from build123d import *

# Parameters (mm, degrees)
BOSS_EXTRUDE1_DEPTH = 2
CUT_EXTRUDE1_DEPTH  = 103
CUT_EXTRUDE2_DEPTH  = 103
SKETCH8_W           = 494.939291997
SKETCH8_H           = 36.91417239
CUT_EXTRUDE3_DEPTH  = 103
SKETCH9_W           = 80
SKETCH9_H           = 22
CUT_EXTRUDE4_DEPTH  = 103
SKETCH10_W          = 80
SKETCH10_H          = 22
CUT_EXTRUDE5_DEPTH  = 10
CUT_EXTRUDE26_DEPTH = 50
SKETCH20_W          = 123.508554763
SKETCH20_H          = 186.038500142
CUT_EXTRUDE27_DEPTH = 50


with BuildPart() as part:
    # Sketch4 → Boss-Extrude1 (new body)
    with BuildSketch(Plane.XY):
        Polygon((-808.497250172, 502.106800376), (-261.98073047, 502.105226222), (-261.98073047, 480.770733626), (-232.677404129, 480.770733626), (-232.677404129, 452.134951617), (-212.25184889, 452.134951617), (-212.192076558, 346.868854324), (-232.677404129, 346.868854324), (-232.677404129, 295.854721303), (-216.917061767, 295.854721303), (-311.499917796, 132.032409135), (-368.546557809, 132.032409135), (-368.546557809, 112.12343356), (-705.513477189, 112.12343356), (-705.513477189, 132.032409135), (-763.511495449, 132.032409135), (-858.513561886, 295.854721303), (-842.744632695, 296.076779874), (-842.744632695, 346.305423028), (-862.968217561, 346.305423028), (-862.968217561, 452.932027611), (-841.983456779, 452.932027611), (-841.983456779, 482.016653843), (-813.304156304, 482.016653843), (-808.497250172, 482.016653843), align=None)
    extrude(amount=BOSS_EXTRUDE1_DEPTH)

    # Sketch6 → Cut-Extrude1 (cut)
    with BuildSketch(Plane.XY.offset(2)):
        Polygon((-822.786730896, 234.247092346), (-802.890229544, 245.785256582), (-762.757484374, 176.580034487), (-782.653985726, 165.041870251), align=None)
    extrude(amount=-CUT_EXTRUDE1_DEPTH, mode=Mode.SUBTRACT)

    # Sketch7 → Cut-Extrude2 (cut)
    with BuildSketch(Plane(origin=(0, 0, 0), x_dir=(-1, 0, 0), z_dir=(0, 0, -1))):
        Polygon((245.988579257, 245.501375956), (264.175112736, 256.001375956), (304.175112736, 186.719343654), (285.988579257, 176.219343654), align=None)
    extrude(amount=-CUT_EXTRUDE2_DEPTH, mode=Mode.SUBTRACT)

    # Sketch8 → Cut-Extrude3 (cut)
    with BuildSketch(Plane.XY.offset(2)):
        with Locations((-533.868102369, 451.361565469)):
            Rectangle(SKETCH8_W, SKETCH8_H)
    extrude(amount=-CUT_EXTRUDE3_DEPTH, mode=Mode.SUBTRACT)

    # Sketch9 → Cut-Extrude4 (cut)
    with BuildSketch(Plane(origin=(0, 0, 0), x_dir=(-1, 0, 0), z_dir=(0, 0, -1))):
        with Locations((427.942047779, 123.12343356)):
            Rectangle(SKETCH9_W, SKETCH9_H)
    extrude(amount=-CUT_EXTRUDE4_DEPTH, mode=Mode.SUBTRACT)

    # Sketch10 → Cut-Extrude5 (cut)
    with BuildSketch(Plane(origin=(0, 0, 0), x_dir=(-1, 0, 0), z_dir=(0, 0, -1))):
        with Locations((644.102693804, 123.12343356)):
            Rectangle(SKETCH10_W, SKETCH10_H)
    extrude(amount=-CUT_EXTRUDE5_DEPTH, mode=Mode.SUBTRACT)

    # Sketch18 → Cut-Extrude26 (cut)
    with BuildSketch(Plane(origin=(0, 0, 0), x_dir=(-1, 0, 0), z_dir=(0, 0, -1))):
        Polygon((232.677404129, 337.860322108), (232.677404129, 496.22384363), (155.712939473, 496.22384363), (155.712939473, 334.151575125), (232.677404129, 334.151575125), align=None)
    extrude(amount=-CUT_EXTRUDE26_DEPTH, mode=Mode.SUBTRACT)

    # Sketch20 → Cut-Extrude27 (cut)
    with BuildSketch(Plane(origin=(0, 0, 0), x_dir=(-1, 0, 0), z_dir=(0, 0, -1))):
        with Locations((903.737734161, 388.997403772)):
            Rectangle(SKETCH20_W, SKETCH20_H)
    extrude(amount=-CUT_EXTRUDE27_DEPTH, mode=Mode.SUBTRACT)


solid = part.part
Source: CAD feature listing. Evaluate the final solid. Frame: model axes, mm. A direction names the side the tool comes from. Round coordinates to 2 decimals unless told otherwise and drop trailing zeros. Loops run counter-clockwise (first coordinate to the right, second up) from the corner with the lowest first, then second, coordinate; pieces in that order, holes last. Notation, with made-up numbers: (59, -18.75) -> (94, -18.75) arc R25 cw to (94, 1.25) -> close; hole circle Ø7 at (11.25, 17). An arc over 180 degrees is marked (long way). Answer as a JSON object with one key per item and string values. Group by question number.
Q1. Section query A-A (y = 459). Output: boundary loops of the cut face in (x, z).
Q2. Mould query, pull axis X, two halves, no side actions, for faces 3 (the flat face through (-812.978, 239.935, 1.014)), 4 (the flat face through (-533, 310, 2)), 5 (the flat face through (-772.57, 170.89, 1.01)). Classes: pulls with the +X half, pulls with the -X half, needs draft (parallel to the pull), parting line crosses it, or undercut.
Q3. Contact query for flat-ended pins moving along their axis: P1, Ø0.6, axis at y = 126, z = 1, coming from the -X side; P2, Ø1, axis at y = 235, z = 1.5, coming from the +X side; P3, Ø0.6, axis at x = -253.5, z = 1.5, coming from the +Y side. Output: stop coordinate, or through.
Q4. Section query C-C (y = 354.5). Output: boundary loops of the cut face in (x, z), plus the area to 3 significant figures.
Q5. Section query B-B (x = -648). Output: boundary loops of the cut face in (y, z), plus the area to 3 significant figures.
Q6. Access query for faces 1 (the flat face through (-840.4, 264.62, 0.99)), 2 (the flat face through (-783.105, 211.667, 1.014)). Directions: +Z, -Z, +X, -X, +Y, -Y. A direction counts if a zero-diameter tool reaches every point of the face in a straight line with its end or side. Return the directions, or none.
Q7. Section query D-D (y = 146.5). Output: boundary loops of the cut face in (x, z).
Q8. Ray query, line 1 (X direction, y = 464, z = 0.9); line 2 (Y direction, x = -690, z = 1.45); line 3 (Y direction, x = -650.5, z = 0.9). Return the intervals inside material, ascending. Write a range as from..to.
Completed:
{
 "1": {"outline": "(-841.98, 0) -> (-781.34, 0) -> (-781.34, 2) -> (-841.98, 2) -> close; (-286.4, 0) -> (-232.68, 0) -> (-232.68, 2) -> (-286.4, 2) -> close"},
 "2": {"face 3": "undercut", "face 4": "needs draft", "face 5": "pulls with the -X half"},
 "3": {"P1": "x = -705.51", "P2": "x = -276.01", "P3": "y = 480.77"},
 "4": {"outline": "(-841.98, 0) -> (-232.68, 0) -> (-232.68, 2) -> (-841.98, 2) -> close", "area": "1,220 mm²"},
 "5": {"outline": "(134.12, 0) -> (432.9, 0) -> (432.9, 2) -> (134.12, 2) -> close; (469.82, 0) -> (502.11, 0) -> (502.11, 2) -> (469.82, 2) -> close", "area": "662 mm²"},
 "6": {"face 1": "+Z, -Z, -X, -Y", "face 2": "+Z, -Z"},
 "7": {"outline": "(-771.9, 0) -> (-303.15, 0) -> (-303.15, 2) -> (-771.9, 2) -> close"},
 "8": {"line 1": "-841.98..-781.34, -286.4..-232.68", "line 2": "112.12..432.9, 469.82..502.11", "line 3": "134.12..432.9, 469.82..502.11"}
}
